The model under review builds one solid part; all positions refer to its coordinate system, in mm. Coordinates: 2 decimals unless noted, no trailing zeros. Write each loop counter-clockwise with the first axis right and the second up, starting at its lowest first coordinate (ties: lowest second). Pieces come first, ordered by that corner, then holes. Notation, with made-up numbers: (46, 69.5) - (96, 69.5) arc R7 cw to (96, 73.5) - close; hole circle Ø3 at (6, -21). An arc over 180 degrees is marked (long way). Return JSON: item names as keys, results as strings. Group by question number.
(1) We need section C-C on z = 1.4. Give the number of separate pieces and of enclosed holes in the cut face, then the cut area to 3 significant figures.
(2) We need section A-A on y = 96.5. State the section outline as (x, z) points, then the cut area to 3 significant figures.
(3) We need section B-B on x = -165.5. State the section outline as (y, z) points, then the cut area to 3 significant figures.
(4) To check wall thickness, follow L1, parallel to Y at x = 31, z = 4.1; L2, parallel to X at y = -141, z = 2.9; L3, parallel to Y at x = 119, z = 3. State the ranges of each line that lie inside material, in increasing order. Write a range as from..to.
(5) For pin 1 Ø1.5 at (y, z) = (96.5, 2.5) entering from +X; pin 2 Ø2.5 at (x, z) = (157.5, 3) entering from +Y; pin 3 Ø2.5 at (x, y) = (20.51, 118.62) entering from -Z; pin 4 Ø2.5 at (x, z) = (157, 2.5) entering from -Y, all flat-tipped, find the tip position at first contact; note any pin that passes through.
```python
from build123d import *

# Parameters (mm, degrees)
SKETCH1_R           = 1.5
SKETCH1_RX          = 129.696010234
SKETCH1_RY          = 100.962749524
BOSS_EXTRUDE1_DEPTH = 5


with BuildPart() as part:
    # Sketch1 → Boss-Extrude1 (new body)
    with BuildSketch(Plane.XY):
        Polygon((155.509699879, -163.878323363), (115.509699879, -163.878323363), (115.509699879, -168.878323363), (85.509699879, -168.878323363), (85.509699879, -163.878323363), (35.509699879, -163.878323363), (35.509699879, -168.878323363), (5.509699879, -168.878323363), (5.509699879, -163.878323363), (-44.490300121, -163.878323363), (-44.490300121, -168.878323363), (-74.490300121, -168.878323363), (-74.490300121, -163.878323363), (-124.490300121, -163.878323363), (-124.490300121, -168.878323363), (-154.490300121, -168.878323363), (-154.490300121, -163.878323363), (-194.490300121, -163.878323363), (-194.490300121, -131.87832215), (-199.490300121, -131.87832215), (-199.490300121, -101.87832215), (-194.490300121, -101.87832215), (-194.490300121, -69.878320937), (-199.490300121, -69.878320937), (-199.490300121, -39.878320937), (-194.490300121, -39.878320937), (-194.490300121, -7.878319723), (-199.490300121, -7.878319723), (-199.490300121, 22.121680277), (-194.490300121, 22.121680277), (-194.490300121, 54.12168149), (-199.490300121, 54.12168149), (-199.490300121, 84.12168149), (-194.490300121, 84.12168149), (-194.490300121, 116.121682703), (-154.490300121, 116.121682703), (-154.490300121, 121.121682703), (-124.490300121, 121.121682703), (-124.490300121, 116.121682703), (-74.490300121, 116.121682703), (-74.490300121, 121.121682703), (-44.490300121, 121.121682703), (-44.490300121, 116.121682703), (5.509699879, 116.121682703), (5.509699879, 121.121682703), (35.509699879, 121.121682703), (35.509699879, 116.121682703), (85.509699879, 116.121682703), (85.509699879, 121.121682703), (115.509699879, 121.121682703), (115.509699879, 116.121682703), (155.509699879, 116.121682703), (155.509699879, 84.12168149), (160.509699879, 84.12168149), (160.509699879, 54.12168149), (155.509699879, 54.12168149), (155.509699879, 22.121680277), (160.509699879, 22.121680277), (160.509699879, -7.878319723), (155.509699879, -7.878319723), (155.509699879, -39.878320937), (160.509699879, -39.878320937), (160.509699879, -69.878320937), (155.509699879, -69.878320937), (155.509699879, -101.87832215), (160.509699879, -101.87832215), (160.509699879, -131.87832215), (155.509699879, -131.87832215), align=None)
        with Locations((-139.490300121, 118.621682703)):
            Circle(SKETCH1_R, mode=Mode.SUBTRACT)
        with Locations((-59.490300121, 118.621682703)):
            Circle(SKETCH1_R, mode=Mode.SUBTRACT)
        with Locations((-196.990300121, 69.12168149)):
            Circle(SKETCH1_R, mode=Mode.SUBTRACT)
        with Locations((-196.990300121, 7.121680277)):
            Circle(SKETCH1_R, mode=Mode.SUBTRACT)
        with Locations(Location((158.009699879, 7.121680277, 0), (0, 0, 180))):
            Circle(SKETCH1_R, mode=Mode.SUBTRACT)
        with Locations(Location((158.009699879, 69.12168149, 0), (0, 0, 180))):
            Circle(SKETCH1_R, mode=Mode.SUBTRACT)
        with Locations(Location((100.509699879, 118.621682703, 0), (0, 0, 180))):
            Circle(SKETCH1_R, mode=Mode.SUBTRACT)
        with Locations(Location((20.509699879, 118.621682703, 0), (0, 0, 180))):
            Circle(SKETCH1_R, mode=Mode.SUBTRACT)
        with Locations((158.009699879, -54.878320937)):
            Circle(SKETCH1_R, mode=Mode.SUBTRACT)
        with Locations((158.009699879, -116.87832215)):
            Circle(SKETCH1_R, mode=Mode.SUBTRACT)
        with Locations((100.509699879, -166.378323363)):
            Circle(SKETCH1_R, mode=Mode.SUBTRACT)
        with Locations((20.509699879, -166.378323363)):
            Circle(SKETCH1_R, mode=Mode.SUBTRACT)
        with Locations(Location((-59.490300121, -166.378323363, 0), (0, 0, 180))):
            Circle(SKETCH1_R, mode=Mode.SUBTRACT)
        with Locations(Location((-139.490300121, -166.378323363, 0), (0, 0, 180))):
            Circle(SKETCH1_R, mode=Mode.SUBTRACT)
        with Locations(Location((-196.990300121, -54.878320937, 0), (0, 0, 180))):
            Circle(SKETCH1_R, mode=Mode.SUBTRACT)
        with Locations(Location((-196.990300121, -116.87832215, 0), (0, 0, 180))):
            Circle(SKETCH1_R, mode=Mode.SUBTRACT)
        with Locations(Location((-19.490300121, -23.87832033), (0, 0, -180))):
            Ellipse(SKETCH1_RX, SKETCH1_RY, mode=Mode.SUBTRACT)
    extrude(amount=BOSS_EXTRUDE1_DEPTH)


solid = part.part
```
Ans:
{
 "1": {"separate pieces": "1", "enclosed holes": "17", "area": "59,100 mm²"},
 "2": {"outline": "(-194.49, 0) - (155.51, 0) - (155.51, 5) - (-194.49, 5) - close", "area": "1,750 mm²"},
 "3": {"outline": "(-163.88, 0) - (116.12, 0) - (116.12, 5) - (-163.88, 5) - close", "area": "1,400 mm²"},
 "4": {"L1": "-168.88..-116.88, 69.12..121.12", "L2": "-194.49..155.51", "L3": "-163.88..116.12"},
 "5": {"pin 1": "x = 155.51", "pin 2": "y = 84.12", "pin 3": "through", "pin 4": "y = -131.88"}
}
